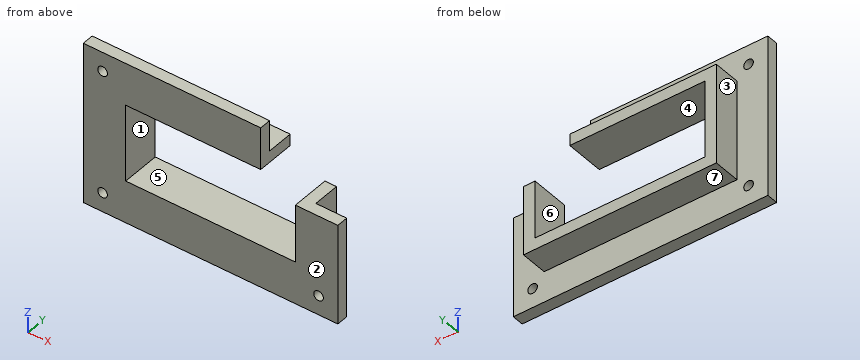
```python
from build123d import *

# Parameters (mm, degrees)
BASE_DEPTH       = 3
WALL_DEPTH       = 7
SKETCH3_R        = 1.25
BOLT_SLOTS_DEPTH = 3


with BuildPart() as part:
    # Sketch1 → base (new body)
    with BuildSketch(Plane(origin=(0, 0, 0), x_dir=(1, 0, 0), z_dir=(0, 1, 0))):
        Polygon((13, -10), (13, -21), (-33, -21), (-33, 21), (33, 21), (33, -5), (22, -5), (22, 10), (-22, 10), (-22, -10), align=None)
    extrude(amount=BASE_DEPTH)

    # Sketch2 → wall (add)
    with BuildSketch(Plane(origin=(0, 3, 0), x_dir=(1, 0, 0), z_dir=(0, 1, 0))):
        Polygon((13, -10), (13, -13), (-25, -13), (-25, 13), (25, 13), (25, -5), (22, -5), (22, 10), (-22, 10), (-22, -10), align=None)
    extrude(amount=WALL_DEPTH)

    # Sketch3 → bolt slots (cut)
    with BuildSketch(Plane(origin=(0, 3, 0), x_dir=(1, 0, 0), z_dir=(0, 1, 0))):
        with Locations(Location((-28, -16, 0), (0, 0, 270))):
            Circle(SKETCH3_R)
        with Locations(Location((-28, 16, 0), (0, 0, 270))):
            Circle(SKETCH3_R)
        with Locations(Location((28, 16, 0), (0, 0, 270))):
            Circle(SKETCH3_R)
    extrude(amount=-BOLT_SLOTS_DEPTH, mode=Mode.SUBTRACT)


solid = part.part
```
Geometry check sheet. Reference: the model listing, model coordinates, mm. Face numbers are marked on the shaded views. A direction names the side the tool comes from. Give positions to 0.01 mm unless a question says otherwise; leave off trailing zeros. Order: outer loops, then holes, each group sorted by start corner. A loop starts at its lowest first (then second) coordinate and runs counter-clockwise, first axis right, second up.
1. Release check for a two-part mould opening along Z. For the marked faces 5, 6 and 7 record: pulls with the +Z half, pulls with the -Z half, needs draft (parallel to the pull), parting line crosses it, or undercut.
2. Section check D-D, the plane y = 2.25. Enter the section's corners in (x, z), and give its area (3 significant figures).
3. Thickness scan on L1, parallel to Z at x = 4.5, y = 4.5; L2, parallel to X at y = 0.95, z = -16; L3, parallel to X at y = 9.5, z = -4.5. Record the ranges inside material, lowest first.
4. Gauge pin test, flat ends, axial feed: pin 1 Ø5.5 at (y, z) = (6.5, -1) entering from +X; pin 2 Ø5 at (y, z) = (7.5, 13.5) entering from +X; pin 3 Ø5.5 at (x, y) = (-11, 6) entering from -Z; pin 4 Ø2 at (x, z) = (28, -16) entering from +Y. Record the tip position at first contact, or that the pin passes through.
5. Access from +Z, -Z, +X, -X, +Y, -Y to the whole of each face (thin tool, end or side, straight path). Record for the marked faces 1, 2, 3 and 4.
6. Section check A-A, the plane z = 16. Enter the section's corners in (x, y).
7. Section check C-C, the plane x = -28. Enter the section's corners in (y, z).
8. Section check B-B, the plane x = 10.5. Enter the section's corners in (y, z).
Values follow:
1. face 5: undercut
1. face 6: needs draft
1. face 7: pulls with the -Z half
2. outline: (-33, -21) - (33, -21) - (33, 5) - (22, 5) - (22, -10) - (-22, -10) - (-22, 10) - (13, 10) - (13, 21) - (-33, 21) - close; hole circle Ø2.5 at (-28, -16); hole circle Ø2.5 at (-28, 16); hole circle Ø2.5 at (28, -16)
2. area: 1,600 mm2
3. L1: z = -13 to -10, 10 to 13
3. L2: x = -33 to -29.25, -26.75 to 26.75, 29.25 to 33
3. L3: x = -25 to -22, 22 to 25
4. pin 1: stops at x = 25
4. pin 2: stops at x = 13
4. pin 3: stops at z = -13
4. pin 4: passes through
5. face 1: +Y, -Y
5. face 2: +Z, -Z, +X, -X, -Y
5. face 3: +Z, -Z, -X, +Y
5. face 4: +X, +Y, -Y
6. outline: (-33, 0) - (-29.25, 0) - (-29.25, 3) - (-33, 3) - close; (-26.75, 0) - (13, 0) - (13, 3) - (-26.75, 3) - close
7. outline: (0, -21) - (3, -21) - (3, -17.25) - (0, -17.25) - close; (0, -14.75) - (3, -14.75) - (3, 14.75) - (0, 14.75) - close; (0, 17.25) - (3, 17.25) - (3, 21) - (0, 21) - close
8. outline: (0, -21) - (3, -21) - (3, -13) - (10, -13) - (10, -10) - (0, -10) - close; (0, 10) - (10, 10) - (10, 13) - (3, 13) - (3, 21) - (0, 21) - close
